```python
from build123d import *

# Parameters (mm, degrees)
SKETCH1_R               = 1.500000001
SKETCH1_R_2             = 1.5
BOSS_EXTRUDE2_DEPTH     = 4
SKETCH1_4_W             = 32
SKETCH1_4_H             = 25
SKETCH1_4_R             = 6.100000001
BOSS_EXTRUDE3_DEPTH     = 20
SKETCH2_R               = 1.5
CUT_EXTRUDE3_DEPTH      = 1
CUT_EXTRUDE3_DEPTH_BACK = 33
CUT_EXTRUDE4_DEPTH      = 5
CUT_EXTRUDE5_START      = -32
CUT_EXTRUDE5_DEPTH      = 5
CUT_EXTRUDE6_DEPTH      = 25
BOSS_EXTRUDE5_DEPTH     = 12.5
CUT_EXTRUDE7_REACH      = 26
SKETCH7_R               = 1.4
BOSS_EXTRUDE6_START     = -32
BOSS_EXTRUDE6_DEPTH     = 10
CUT_EXTRUDE8_DEPTH      = 43


with BuildPart() as part:
    # Sketch1 → Boss-Extrude2 (new body)
    with BuildSketch(Plane.XY):
        Polygon((-16, 39), (-16, -46.5), (-14.969293645, -46.5), (-14.969293645, -42.160880121), (-15.92820323, -40.5), (-12.464101615, -34.5), (-5.535898385, -34.5), (-2.07179677, -40.5), (-5.535898385, -46.5), (5.535898385, -46.5), (2.090853862, -40.533007852), (5.457729166, -34.432863746), (12.425340481, -34.432863746), (15.909146138, -40.466992148), (15, -42.114193768), (15, -46.5), (16, -46.5), (16, 39), align=None)
        with Locations((10, 10)):
            Circle(SKETCH1_R, mode=Mode.SUBTRACT)
        with Locations((-10, -10)):
            Circle(SKETCH1_R, mode=Mode.SUBTRACT)
        with Locations((10, -10)):
            Circle(SKETCH1_R, mode=Mode.SUBTRACT)
        with Locations((-10, 10)):
            Circle(SKETCH1_R, mode=Mode.SUBTRACT)
        with Locations((0, -43.5)):
            Circle(SKETCH1_R_2, mode=Mode.SUBTRACT)
        with Locations((-8.5, -31.5)):
            Circle(SKETCH1_R_2, mode=Mode.SUBTRACT)
        with Locations((8.5, -31.5)):
            Circle(SKETCH1_R_2, mode=Mode.SUBTRACT)
    extrude(amount=BOSS_EXTRUDE2_DEPTH)

    # Sketch1<4> → Boss-Extrude3 (add)
    with BuildSketch(Plane.XY):
        with Locations((0, 26.5)):
            Rectangle(SKETCH1_4_W, SKETCH1_4_H)
        Polygon((0, 36.969655115), (9.5, 31.484827557), (9.5, 20.515172443), (0, 15.030344885), (-9.5, 20.515172443), (-9.5, 31.484827557), align=None, mode=Mode.SUBTRACT)
        Polygon((9.5, 31.484827557), (9.5, 20.515172443), (0, 15.030344885), (-9.5, 20.515172443), (-9.5, 31.484827557), (0, 36.969655115), align=None)
        with Locations((0, 26)):
            Circle(SKETCH1_4_R, mode=Mode.SUBTRACT)
        with Locations((0, 26)):
            Circle(SKETCH1_4_R)
    extrude(amount=-BOSS_EXTRUDE3_DEPTH)

    # Sketch2 → Cut-Extrude3 (cut, two sides)
    with BuildSketch(Plane.ZY.offset(16)) as cut_extrude3_sk:
        with Locations((-1.580023732, 25.999827557)):
            Circle(SKETCH2_R)
    extrude(amount=CUT_EXTRUDE3_DEPTH, mode=Mode.SUBTRACT)
    extrude(cut_extrude3_sk.sketch, amount=-CUT_EXTRUDE3_DEPTH_BACK, mode=Mode.SUBTRACT)

    # Sketch3 → Cut-Extrude4 (cut)
    with BuildSketch(Plane.ZY.offset(16)):
        with BuildLine():
            Line((0.716979622, 28.369168308), (-1.239134605, 30.265561192))
            ThreePointArc((-1.239134605, 30.265561192), (-1.539975782, 30.904899692), (-1.343104133, 31.583501701))
            ThreePointArc((-1.343104133, 31.583501701), (0.822230527, 35.120419324), (2.287602236, 39))
            Line((2.287602236, 39), (-20, 39))
            Line((-20, 39), (-20, 22.778106647))
            ThreePointArc((-20, 22.778106647), (-13.472070231, 23.458477945), (-7.432949471, 26.028651597))
            ThreePointArc((-7.432949471, 26.028651597), (-6.799957072, 26.171029415), (-6.212814046, 25.894960789))
            Line((-6.212814046, 25.894960789), (-3.877027086, 23.630486807))
            Line((-3.877027086, 23.630486807), (0.716979622, 28.369168308))
        make_face()
        with BuildLine():
            ThreePointArc((-3.877027086, 23.630486807), (0.789317018, 23.702824203), (0.716979622, 28.369168308))
            Line((0.716979622, 28.369168308), (-3.877027086, 23.630486807))
        make_face()
    extrude(amount=-CUT_EXTRUDE4_DEPTH, mode=Mode.SUBTRACT)

    # Sketch3<4> → Cut-Extrude5 (cut)
    with BuildSketch(Plane.ZY.offset(16).offset(CUT_EXTRUDE5_START)):
        with BuildLine():
            Line((0.716979622, 28.369168308), (-1.239134605, 30.265561192))
            ThreePointArc((-1.239134605, 30.265561192), (-1.539975782, 30.904899692), (-1.343104133, 31.583501701))
            ThreePointArc((-1.343104133, 31.583501701), (0.822230527, 35.120419324), (2.287602236, 39))
            Line((2.287602236, 39), (-20, 39))
            Line((-20, 39), (-20, 22.778106647))
            ThreePointArc((-20, 22.778106647), (-13.472070231, 23.458477945), (-7.432949471, 26.028651597))
            ThreePointArc((-7.432949471, 26.028651597), (-6.799957072, 26.171029415), (-6.212814046, 25.894960789))
            Line((-6.212814046, 25.894960789), (-3.877027086, 23.630486807))
            Line((-3.877027086, 23.630486807), (0.716979622, 28.369168308))
        make_face()
        with BuildLine():
            ThreePointArc((-3.877027086, 23.630486807), (0.789317018, 23.702824203), (0.716979622, 28.369168308))
            Line((0.716979622, 28.369168308), (-3.877027086, 23.630486807))
        make_face()
    extrude(amount=CUT_EXTRUDE5_DEPTH, mode=Mode.SUBTRACT)

    # Sketch5 → Cut-Extrude6 (cut, through all)
    with BuildSketch(Plane.XY.offset(4)):
        Polygon((-14.969293645, -42.160880121), (-15.92820323, -40.5), (-16, -40.500074436), (-16, -46.5), (-14.969293645, -46.5), align=None)
        Polygon((15, -42.114193768), (15.909146138, -40.466992148), (10.36687247, -40.472738184), (10.36687247, -46.5), (15, -46.5), align=None)
        Polygon((16, -40.466897954), (15.909146138, -40.466992148), (15, -42.114193768), (15, -46.5), (16, -46.5), align=None)
        Polygon((17.825288522, -40.465005559), (16, -40.466897954), (16, -46.5), (17.916172301, -46.5), align=None)
    extrude(amount=-CUT_EXTRUDE6_DEPTH, mode=Mode.SUBTRACT)

    # Sketch8 → Boss-Extrude5 (add)
    with BuildSketch(Plane.ZY.offset(16)):
        with BuildLine():
            ThreePointArc((-1.343104133, 31.583501701), (-1.539975782, 30.904899692), (-1.239134605, 30.265561192))
            Line((-1.239134605, 30.265561192), (0.716979622, 28.369168308))
            ThreePointArc((0.716979622, 28.369168308), (0.789317018, 23.702824203), (-3.877027086, 23.630486807))
            Line((-3.877027086, 23.630486807), (-6.212814046, 25.894960789))
            ThreePointArc((-6.212814046, 25.894960789), (-6.799957072, 26.171029415), (-7.432949471, 26.028651597))
            ThreePointArc((-7.432949471, 26.028651597), (-13.472070231, 23.458477945), (-20, 22.778106647))
            Line((-20, 22.778106647), (-20, 14))
            Line((-20, 14), (0, 14))
            Line((0, 14), (4, 14))
            Line((4, 14), (4, 39))
            Line((4, 39), (2.287602236, 39))
            ThreePointArc((2.287602236, 39), (0.822230527, 35.120419324), (-1.343104133, 31.583501701))
        make_face()
    extrude(amount=BOSS_EXTRUDE5_DEPTH)

    # Sketch7 → Cut-Extrude7 (cut, up to next)
    with BuildSketch(Plane.XY.offset(4), mode=Mode.PRIVATE) as cut_extrude7_sk1:
        with Locations((-23.5, 27.75)):
            Circle(SKETCH7_R)
    cut_extrude7_tool1 = extrude(cut_extrude7_sk1.sketch, amount=-CUT_EXTRUDE7_REACH, mode=Mode.PRIVATE) & part.part
    add(cut_extrude7_tool1.solids().sort_by_distance((-23.5, 27.75, 4))[0], mode=Mode.SUBTRACT)
    # Sketch7 → Cut-Extrude7 (cut, up to next)
    with BuildSketch(Plane.XY.offset(4), mode=Mode.PRIVATE) as cut_extrude7_sk2:
        with Locations((-13.5, 27.75)):
            Circle(SKETCH7_R)
    cut_extrude7_tool2 = extrude(cut_extrude7_sk2.sketch, amount=-CUT_EXTRUDE7_REACH, mode=Mode.PRIVATE) & part.part
    add(cut_extrude7_tool2.solids().sort_by_distance((-13.5, 27.75, 4))[0], mode=Mode.SUBTRACT)

    # Sketch8<3> → Boss-Extrude6 (add)
    with BuildSketch(Plane.ZY.offset(16).offset(BOSS_EXTRUDE6_START)):
        with BuildLine():
            ThreePointArc((-1.343104133, 31.583501701), (-1.539975782, 30.904899692), (-1.239134605, 30.265561192))
            Line((-1.239134605, 30.265561192), (0.716979622, 28.369168308))
            ThreePointArc((0.716979622, 28.369168308), (0.789317018, 23.702824203), (-3.877027086, 23.630486807))
            Line((-3.877027086, 23.630486807), (-6.212814046, 25.894960789))
            ThreePointArc((-6.212814046, 25.894960789), (-6.799957072, 26.171029415), (-7.432949471, 26.028651597))
            ThreePointArc((-7.432949471, 26.028651597), (-13.472070231, 23.458477945), (-20, 22.778106647))
            Line((-20, 22.778106647), (-20, 14))
            Line((-20, 14), (0, 14))
            Line((0, 14), (4, 14))
            Line((4, 14), (4, 39))
            Line((4, 39), (2.287602236, 39))
            ThreePointArc((2.287602236, 39), (0.822230527, 35.120419324), (-1.343104133, 31.583501701))
        make_face()
    extrude(amount=-BOSS_EXTRUDE6_DEPTH)

    # Sketch8<4> → Cut-Extrude8 (cut, through all)
    with BuildSketch(Plane.ZY.offset(16)):
        with BuildLine():
            ThreePointArc((-1.343104133, 31.583501701), (-4.126373378, 28.519223025), (-7.432949471, 26.028651597))
            ThreePointArc((-7.432949471, 26.028651597), (-13.472070231, 23.458477945), (-20, 22.778106647))
            Line((-20, 22.778106647), (-20, 39))
            Line((-20, 39), (2.287602236, 39))
            ThreePointArc((2.287602236, 39), (0.822230527, 35.120419324), (-1.343104133, 31.583501701))
        make_face()
    extrude(amount=-CUT_EXTRUDE8_DEPTH, mode=Mode.SUBTRACT)


solid = part.part
```
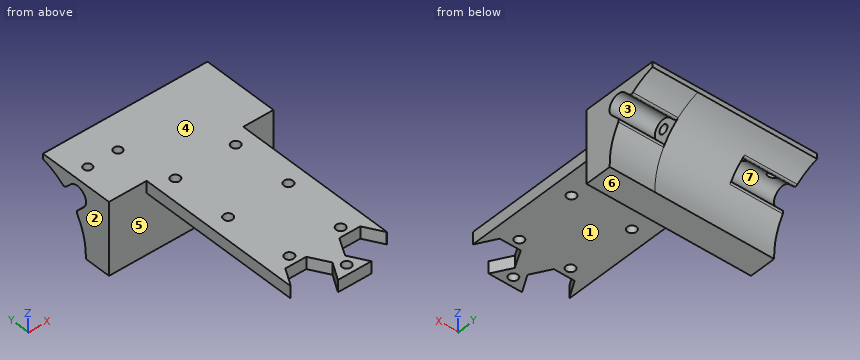
The listing builds one solid part. Answer for the finished solid, in the listing's coordinates (mm). Face numbers are marked on the shaded views. A direction names the side the tool comes from. Round coordinates to 2 decimals unless told otherwise and drop trailing zeros. Loops run counter-clockwise (first coordinate to the right, second up) from the corner with the lowest first, then second, coordinate; pieces in that order, holes last. Notation, with made-up numbers: (-3.75, -32.5) - (17.25, -32.5) arc R25 ccw to (17.25, 5.5) - close; hole circle Ø2 at (7.25, 81). An arc over 180 degrees is marked (long way). Use one line per item in the form item = value. Start each with the question number.
1. Given pin 1 Ø7 at (x, z) = (7.5, -11.5) entering from -Y; pin 2 Ø1.2 at (x, z) = (-10, 1) entering from -Y; pin 3 Ø8 at (x, z) = (20, -0.5) entering from +Y; pin 4 Ø1.2 at (y, z) = (-23, 1) entering from -X, each flat-ended and moving along its own axis, determine where each tip first touches the part or whether it passes through.
2. The part is cut by section B-B on y = -36. Determine the outline of the cut face in (x, z), then the cut area to 3 significant figures.
3. A tool of negligible diameter and unlimited length cuts with its end or side. For the marked faces 1, 2 and 3, from which of +Z, -Z, +X, -X, +Y, -Y can it reach the whole face along a straight path? Write none if from no direction.
4. Consider line 1 (X direction, y = 27.75, z = 1.6); line 2 (Y direction, x = -23.5, z = 2.9); line 3 (Z direction, x = -1, y = -11). Determine where each line is inside the solid, lowest interval first. Write a range as [from, to].
5. For a pull along Z with two mould halves and no side action, classify the marked faces 4, 5, 6 and 7 as pulls with the +Z half, pulls with the -Z half, needs draft (parallel to the pull), parting line crosses it, or undercut.
6. The part is cut by section A-A on x = 0. Determine the outline of the cut face in (y, z), then the cut area to 3 significant figures.
7. The part is cut by section C-C on x = 21. Determine the outline of the cut face in (y, z), then the cut area to 3 significant figures.
8. The part is cut by section D-D on x = -13.5. Determine the outline of the cut face in (y, z).
Geometry check:
q1.pin_1 = 14
q1.pin_2 = -34.5
q1.pin_3 = 39
q1.pin_4 = -16
q2.outline = (-16, 0) - (-13.33, 0) - (-13.33, 4) - (-16, 4) - close; (-4.67, 0) - (4.59, 0) - (4.59, 4) - (-4.67, 4) - close; (13.33, 0) - (16, 0) - (16, 4) - (13.33, 4) - close
q2.area = 58.4 mm^2
q3.face_1 = -Z, +X, -X, -Y
q3.face_2 = +Z, -Z, -X, +Y, -Y
q3.face_3 = +X
q4.line_1 = [-28.5, -24.9], [-22.1, -14.9], [-12.1, 26]
q4.line_2 = [14, 26.35], [29.15, 39]
q4.line_3 = [0, 4]
q5.face_4 = pulls with the +Z half
q5.face_5 = needs draft
q5.face_6 = pulls with the -Z half
q5.face_7 = undercut
q6.outline = (-46.5, 0) - (-45, 0) - (-45, 4) - (-46.5, 4) - close; (-42, 0) - (14, 0) - (14, -20) - (22.78, -20) arc R22.07 cw to (39, 2.29) - (39, 4) - (-42, 4) - close; hole circle Ø3 at (26, -1.58)
q6.area = 551 mm^2
q7.outline = (14, -20) - (22.78, -20) arc R22.07 cw to (26.03, -7.43) arc R1 ccw to (25.89, -6.21) - (23.63, -3.88) arc R3.3 cw to (28.37, 0.72) - (30.27, -1.24) arc R1 ccw to (31.58, -1.34) arc R22.07 cw to (39, 2.29) - (39, 4) - (14, 4) - close
q7.area = 287 mm^2
q8.outline = (-36.29, 0) - (14, 0) - (14, -20) - (22.78, -20) arc R22.07 cw to (26.03, -7.43) arc R1 ccw to (25.89, -6.21) - (23.63, -3.88) arc R3.3 cw to (26.35, 1.7) - (26.35, 4) - (-36.29, 4) - close; (29.15, -0.09) - (30.27, -1.24) arc R1 ccw to (31.58, -1.34) arc R22.07 cw to (39, 2.29) - (39, 4) - (29.15, 4) - close
